Geometry: final body of the model. Coordinates: model frame, mm. A direction names the side the tool comes from. Give positions to 0.01 mm unless a question says otherwise; leave off trailing zeros. Loops run counter-clockwise (first coordinate to the right, second up) from the corner with the lowest first, then second, coordinate; pieces in that order, holes last.
from build123d import *

# Parameters (mm, degrees)
F0_R     = 12.5
F0_R_2   = 2.15
F0_W     = 3
F0_H     = 6
F1_DEPTH = 6
F0_R_3   = 1.65
F2_DEPTH = 1
F3_R     = 1.75
F4_DEPTH = 12.5
F5_START = 10
F3_R_2   = 3.2
F5_DEPTH = 15


with BuildPart() as f1:
    # F0 (on Top) → F1 (new body)
    with BuildSketch(Plane.XY):
        Circle(F0_R)
        with Locations((0, -9)):
            Circle(F0_R_2, mode=Mode.SUBTRACT)
        with BuildLine():
            ThreePointArc((-1.5, 2.1052850163), (1.1842138743, 2.2977951388), (2.585, 0))
            ThreePointArc((2.585, 0), (1.1842138743, -2.2977951388), (-1.5, -2.1052850163))
            ThreePointArc((-1.5, -2.1052850163), (-2.585, 0), (-1.5, 2.1052850163))
        make_face(mode=Mode.SUBTRACT)
        with Locations((6, 0)):
            Rectangle(F0_W, F0_H, mode=Mode.SUBTRACT)
        with Locations((0, 9)):
            Circle(F0_R_2, mode=Mode.SUBTRACT)
        with BuildLine():
            Line((-1.5, -2.1052850163), (-1.5, 2.1052850163))
            ThreePointArc((-1.5, 2.1052850163), (-2.585, 0), (-1.5, -2.1052850163))
        make_face()
    extrude(amount=F1_DEPTH)

    # F0 (on Top) → F2 (join)
    with BuildSketch(Plane.XY):
        with Locations((0, 9)):
            Circle(F0_R_2)
        with Locations((0, 9)):
            Circle(F0_R_3, mode=Mode.SUBTRACT)
        with Locations((0, -9)):
            Circle(F0_R_2)
        with Locations((0, -9)):
            Circle(F0_R_3, mode=Mode.SUBTRACT)
    extrude(amount=F2_DEPTH)

    # F3 (on Right) → F4 (cut, symmetric)
    with BuildSketch(Plane.YZ):
        with Locations((0, 3)):
            Circle(F3_R)
    extrude(amount=F4_DEPTH, both=True, mode=Mode.SUBTRACT)

    # F3 (on Right) → F5 (cut)
    with BuildSketch(Plane.YZ.offset(F5_START)):
        with Locations((0, 3)):
            Circle(F3_R_2)
        with Locations((0, 3)):
            Circle(F3_R, mode=Mode.SUBTRACT)
    extrude(amount=F5_DEPTH, mode=Mode.SUBTRACT)


solid = f1.part
Item 1: Section query D-D on y = -9. Return loops of the section in (x, z), plus the area to 3 significant figures.
Values follow:
outline: (-8.67, 0) - (-1.65, 0) - (-1.65, 1) - (-2.15, 1) - (-2.15, 6) - (-8.67, 6) - close; (1.65, 0) - (8.67, 0) - (8.67, 6) - (2.15, 6) - (2.15, 1) - (1.65, 1) - close
area: 79.3 mm2
Item 2: Section query C-C on x = 7. Return loops of the section in (y, z).
Values follow:
outline: (-10.36, 0) - (-3, 0) - (-3, 6) - (-10.36, 6) - close; (3, 0) - (10.36, 0) - (10.36, 6) - (3, 6) - close
Item 3: Section query A-A on z = 3.5. Return loops of the section in (x, y) (3 decimals).
Values follow:
outline: (-12.387, -1.677) arc R12.5 ccw to (12.094, -3.161) - (10, -3.161) - (10, -1.677) - (7.5, -1.677) - (7.5, -3) - (4.5, -3) - (4.5, -1.677) - (1.967, -1.677) arc R2.585 cw to (-1.5, -2.105) - (-1.5, -1.677) - close; (-12.387, 1.677) - (-1.5, 1.677) - (-1.5, 2.105) arc R2.585 cw to (1.967, 1.677) - (4.5, 1.677) - (4.5, 3) - (7.5, 3) - (7.5, 1.677) - (10, 1.677) - (10, 3.161) - (12.094, 3.161) arc R12.5 ccw to start; hole circle Ø4.3 at (0, -9); hole circle Ø4.3 at (0, 9)
Item 4: Draft query along X for faces 1 (the face through (10, 1.4, 4.4)), 2 (the face through (6, 3, 3)), 3 (the face through (-3, 0, 6)). Return one class per face: +X half, -X half, draft (parallel to the pull), parting line (faces both ways), or undercut.
Values follow:
face 1: +X half
face 2: undercut
face 3: draft
Item 5: Ray query, probe 1 along Y at (x, z) = (0, 0.5) (3 decimals); probe 2 along Z at (x, y) = (2.75, 0); probe 3 along Y at (x, z) = (-1.75, 5). Return the intervals inside material, ascending.
Values follow:
probe 1: y = -12.5 to -10.65, -7.35 to -2.585, 2.585 to 7.35, 10.65 to 12.5
probe 2: z = 0 to 1.25, 4.75 to 6
probe 3: y = -12.38 to -10.25, -7.75 to 7.75, 10.25 to 12.38
Item 6: Section query B-B on x = 0. Return loops of the section in (y, z) (3 decimals), plus the area to 3 significant figures.
Values follow:
outline: (-12.5, 0) - (-10.65, 0) - (-10.65, 1) - (-11.15, 1) - (-11.15, 6) - (-12.5, 6) - close; (-7.35, 0) - (-2.585, 0) - (-2.585, 6) - (-6.85, 6) - (-6.85, 1) - (-7.35, 1) - close; (2.585, 0) - (7.35, 0) - (7.35, 1) - (6.85, 1) - (6.85, 6) - (2.585, 6) - close; (10.65, 0) - (12.5, 0) - (12.5, 6) - (11.15, 6) - (11.15, 1) - (10.65, 1) - close
area: 69.4 mm2
Item 7: Set-up query: faces 4 (the face through (-1.5, -1.9, 2.96)), 5 (the face through (11.2, -3.2, 3.1)), 6 (the face through (8.77, -0.38, 1.29)), 7 (the face through (0, -3, 0)), 8 (the face through (0, 7, 1)). Return all of +Z, -Z, +X, -X, +Y, -Y with unobstructed straight access to the full face (end or side cutting, diameter ignored); none if empty.
Values follow:
face 4: +Z, -Z
face 5: +X
face 6: +X, -X
face 7: -Z, +X, -X, +Y, -Y
face 8: +Z
Item 8: Pin query (flat end, axial travel): pin 1 (1.5 mm diameter, centred on x = 5.5, z = 4, fed in from +Y); pin 2 (2.5 mm diameter, centred on x = 6, z = 3, fed in from -Y); pin 3 (3.5 mm diameter, centred on x = 0, y = -10, fed in from +Z); pin 4 (3.5 mm diameter, centred on y = -0.5, z = 3, fed in from +X). Return the tip coordinate at first contact, or that it passes through.
Values follow:
pin 1: stops at y = 11.56
pin 2: stops at y = -11.56
pin 3: stops at z = 6
pin 4: stops at x = 10
